Here's the drawing with two shaded views (mm, measured from the low corner). I have some questions. Round coordinates to 2 decimals unless told otherwise and drop trailing zeros. Order: outer loops, then holes, each group sorted by start corner. A loop starts at its lowest first (then second) coordinate and runs counter-clockwise, first axis right, second up. Notation, with made-up numbers: (23, -35.5) -> (63, -35.5) arc R22 ccw to (63, -2.5) -> close; hole circle Ø2 at (0.5, 71). An arc over 180 degrees is marked (long way). One line per question, with ' | ' between items.
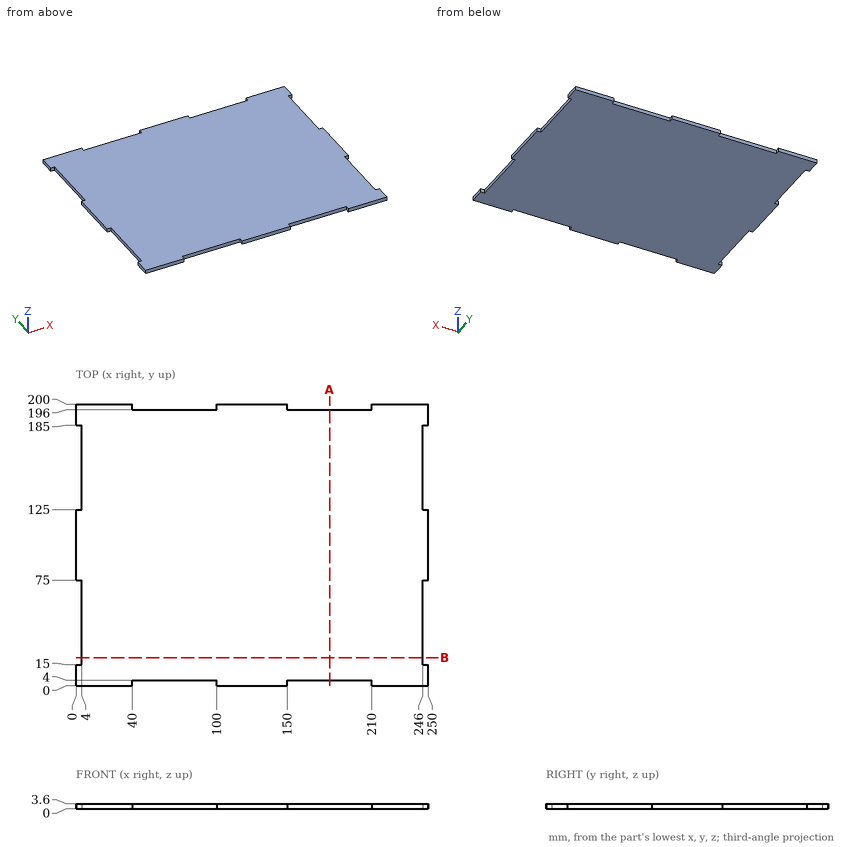
1. I want a section at B-B on y = 20. List the corners of the cut face in (x, z) for me, and give its area (3 significant figures).
From the geometry:
outline: (4, 0) -> (246, 0) -> (246, 3.6) -> (4, 3.6) -> close | area: 871 mm²
2. I want a section at A-A on x = 180. List the corners of the cut face in (y, z) for me.
From the geometry:
outline: (4, 0) -> (196, 0) -> (196, 3.6) -> (4, 3.6) -> close
3. I'm going to push flat-ended pins straight in: pin 1 (1.5 mm diameter, centred on x = 127.5, y = 73.5, fed in from -Z); pin 2 (1.8 mm diameter, centred on y = 42, z = 2, fed in from +X); pin 3 (1.8 mm diameter, centred on x = 83, z = 1, fed in from +Y). Where does each tip first touch, or does it pass through?
From the geometry:
pin 1: stops at z = 0 | pin 2: stops at x = 246 | pin 3: stops at y = 196
4. I need wall thicknesses on probe 1 along X at (y, z) = (145, 3.3); probe 2 along Y at (x, z) = (52.5, 3.35). Which ranges of each line are inside material? Lowest first, please.
From the geometry:
probe 1: x = 4 to 246 | probe 2: y = 4 to 196
